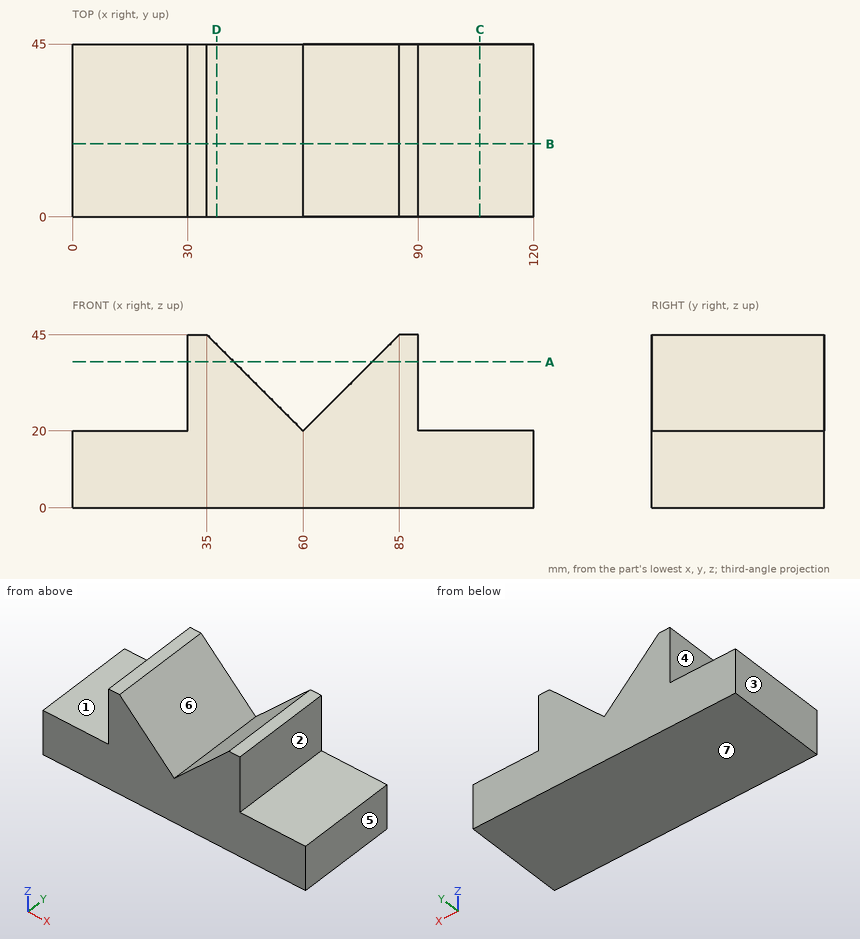
Verification items for this drawing (mm, ordinates from the low corner). A direction names the side the tool comes from. Coordinates: 2 decimals unless noted, no trailing zeros. Order: outer loops, then holes, each group sorted by start corner. A loop starts at its lowest first (then second) coordinate and runs counter-clockwise, first axis right, second up. Notation, with made-up numbers: (72, 5.5) - (83, 5.5) arc R9 cw to (83, 19.5) - close; hole circle Ø5 at (36.25, 3.5). An arc over 180 degrees is marked (long way). Answer in a Markdown table with one row per item. Add a question column.
1. Section check B-B (y = 19). Enter the section's corners in (x, z).
2. Section check C-C (x = 106). Enter the section's corners in (y, z), plus the area to 3 significant figures.
3. Section check A-A (z = 38). Enter the section's corners in (x, y).
4. Gauge pin test, flat ends, axial feed: pin 1 Ø9 at (x, y) = (15, 15) entering from +Z; pin 2 Ø5 at (y, z) = (22.5, 26) entering from +X. Record the tip position at first contact, or that the pin passes through.
5. Draft check along X on the marked faces 4, 5, 6 and 7. Enter one of: +X half, -X half, draft (parallel to the pull), parting line (faces both ways), or undercut.
6. Section check D-D (x = 37.5). Enter the section's corners in (y, z), plus the area to 3 significant figures.
7. Access from +Z, -Z, +X, -X, +Y, -Y to the whole of each face (thin tool, end or side, straight path). Record for the marked faces 1, 2 and 3.
8. Material ranges on L1, parallel to Z at x = 18, y = 20.5; L2, parallel to X at y = 39, z = 35.5; L3, parallel to X at y = 41, z = 37, recorded low to high. Write a range as [from, to].
Data:
| question | item | result |
|---|---|---|
| 1 | outline | (0, 0) - (120, 0) - (120, 20) - (90, 20) - (90, 45) - (85, 45) - (60, 20) - (35, 45) - (30, 45) - (30, 20) - (0, 20) - close |
| 2 | outline | (0, 0) - (45, 0) - (45, 20) - (0, 20) - close |
| 2 | area | 900 mm² |
| 3 | outline | (30, 0) - (42, 0) - (42, 45) - (30, 45) - close; (78, 0) - (90, 0) - (90, 45) - (78, 45) - close |
| 4 | pin 1 | stops at z = 20 |
| 4 | pin 2 | stops at x = 90 |
| 5 | face 4 | -X half |
| 5 | face 5 | +X half |
| 5 | face 6 | undercut |
| 5 | face 7 | draft |
| 6 | outline | (0, 0) - (45, 0) - (45, 42.5) - (0, 42.5) - close |
| 6 | area | 1,910 mm² |
| 7 | face 1 | +Z, -X, +Y, -Y |
| 7 | face 2 | +Z, +X, +Y, -Y |
| 7 | face 3 | +Z, -Z, -X, +Y, -Y |
| 8 | L1 | z = [0, 20] |
| 8 | L2 | x = [30, 44.5], [75.5, 90] |
| 8 | L3 | x = [30, 43], [77, 90] |
